Autodesk Inventor part; units mm, degrees
ref_plane "YZ Plane" through (0, 0, 0) normal (1, 0, 0) x (0, 1, 0)
ref_plane "XZ Plane" through (0, 0, 0) normal (0, 1, 0) x (-1, 0, 0)
ref_plane "XY Plane" through (0, 0, 0) normal (0, 0, 1) x (1, 0, 0)
sketch "スケッチ1" plane through (0, 0, 0) normal (0, 0, 1) x (1, 0, 0)
  circle A0 centre (0, 0) radius 13.5
  line L0 (0, 13.5) -> (14.5, 13.5)
  line L1 (14.5, 13.5) -> (14.5, -13.5)
  line L2 (14.5, -13.5) -> (0, -13.5)
  line L3 (0, -13.5) -> (0, 13.5)
  line L4 (0, 0) -> (14.5, 0) construction
  point P0 (0, 13.5)
  point P1 (0, -13.5)
  point P2 (0, -13.5)
  dimension "d0" = 27
  dimension "d1" = 27
  dimension "d2" = 14.5
extrude "プレート1" add sketch "スケッチ1" along normal blind 3
sketch "スケッチ2" plane through (17.5, 13.5, 6) normal (1, 0, 0) x (0, 1, 0)
  line L0 (-27, 0) -> (0, 0)
  line L1 (0, 0) -> (0, 19)
  line L2 (0, 19) -> (-27, 19)
  line L3 (-27, 19) -> (-27, 0)
edge flange "フランジ1" height 25 angle 90 thickness 3 bend radius 3 thickness toward (1, 0, 0) relief tear relief width 3 relief depth 1.5 edges at (14.5, 0, 3) wall of the first edge with corners at (17.5, -13.5, 6) (17.5, 13.5, 6) (17.5, 13.5, 25) (17.5, -13.5, 25)
bend "曲げ1"
corner "コーナー1"
sketch "スケッチ3" plane through (0, 0, 0) normal (0, 0, -1) x (-1, 0, 0)
  point P0 (0, 0)
  point P1 (10, 0)
  point P2 (-5, 8.6603)
  point P3 (-5, -8.6603)
  dimension "d14" = 10
  dimension "d17" = 360
hole "穴1" at (-10, 0, 0) at (5, 8.6603, 0) at (5, -8.6603, 0) direction (0, 0, 1) diameter 2.7 depth 3
sketch "スケッチ4" plane through (20.5, -13.5, 25) normal (1, 0, 0) x (0, 0, -1)
  circle A0 centre (-2, 14.5) radius 21
  line L0 (25, 27) -> (25, 0)
  point P0 (25, 13.5)
  dimension "d26" = 42
  dimension "d29" = 27
extrude "押し出し1" add sketch "スケッチ4" against normal up to surface (3 mm away)
sketch "スケッチ5" plane through (20.5, -13.5, 6) normal (1, 0, 0) x (0, 0, -1)
  arc A0 (-4.1255, 27) -> (-5.8095, 0) centre (-21, 14.5) ccw
  circle A1 centre (-21, 14.5) radius 14.5
  point P0 (6, 13.5)
  dimension "d30" = 29
extrude "押し出し2" cut sketch "スケッチ5" against normal up to surface (3 mm away)
sketch "スケッチ7" plane through (20.5, -13.5, 6) normal (1, 0, 0) x (0, 0, -1)
  circle A0 centre (-21, 14.5) radius 14.5
  point P0 (6, 13.5)
  point P1 (-39.5, 14.5)
  point P2 (-11.75, -1.5215)
  point P3 (-11.75, 30.5215)
  dimension "d33" = 18.5
  dimension "d36" = 360
hole "穴2" at (20.5, 1, 45.5) at (20.5, -15.0215, 17.75) at (20.5, 17.0215, 17.75) direction (-1, 0, 0) diameter 2.7 depth 3
fillet "フィレット1" radius 10 2 edges at (19, -13.5, 11.8095) (19, 13.5, 10.1255)
sketch "スケッチ9" plane through (0, 0, 0) normal (0, 0, -1) x (-1, 0, 0)
  arc A0 (0, -13.5) -> (0, 13.5) centre (0, 0) ccw
  line L0 (0, 13.5) -> (13.5, 13.5)
  line L1 (13.5, 13.5) -> (13.5, -13.5)
  line L2 (13.5, -13.5) -> (0, -13.5)
  line L3 (0, -13.5) -> (0, 13.5)
  circle A1 centre (-5, -8.6603) radius 1.35
  circle A2 centre (-5, 8.6603) radius 1.35
  circle A3 centre (10, 0) radius 1.35
  line L4 (0, 13.5) -> (-14.5, 13.5)
  line L5 (-14.5, 13.5) -> (-14.5, -13.5)
  line L6 (-14.5, -13.5) -> (0, -13.5)
  arc A4 (0, -13.5) -> (0, 13.5) centre (0, 0) ccw
  point P0 (13.5, 0)
  dimension "d48" = 13.5
  dimension "d49" = 27
extrude "押し出し3" add sketch "スケッチ9" against normal up to surface (3 mm away) contours A0 L1 L2 | A0 L0 L1
fillet "フィレット2" radius 6 2 edges at (-13.5, 13.5, 1.5) (-13.5, -13.5, 1.5)
equation "\"d24\" = Thickness"
equation "\"d3\" = Thickness"
equation "\"d4\" = BendReliefWidth"
equation "\"d5\" = BendReliefDepth"
equation "\"d6\" = MinimumRemnant"
equation "\"d7\" = TransitionRadius"
equation "\"d10\" = BendRadius"
equation "\"d11\" = CornerReliefSize"
equation "\"d12\" = GapSize"
equation "\"d13\" = JacobiRadiusSize"
equation "\"BendRadius\" = Thickness"
equation "\"BendReliefWidth\" = Thickness"
equation "\"BendReliefDepth\" = 0.5 * Thickness"
equation "\"CornerReliefSize\" = 4 * Thickness"
equation "\"MinimumRemnant\" = 2 * Thickness"
equation "\"TransitionRadius\" = BendRadius"
equation "\"JacobiRadiusSize\" = BendRadius"
equation "\"GapSize\" = Thickness"
properties part number "wrist_roll_plate" material "アルミニウム 6061"
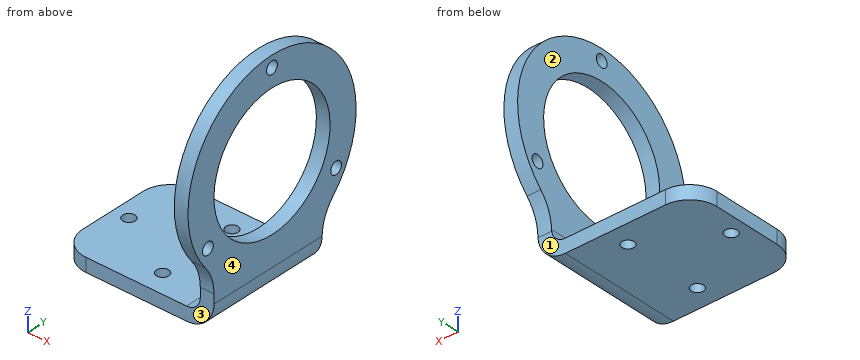
Source: CAD feature listing. Evaluate the final solid. Frame: model axes, mm. Face numbers are marked on the shaded views. A direction names the side the tool comes from. Round coordinates to 2 decimals unless told otherwise and drop trailing zeros. Loops run counter-clockwise (first coordinate to the right, second up) from the corner with the lowest first, then second, coordinate; pieces in that order, holes last. Notation, with made-up numbers: (75, 20) - (121, 20) arc R7 cw to (121, 30) - close; hole circle Ø9 at (-40, 6.25). An arc over 180 degrees is marked (long way). Write item = value, one per line. Start each with the question number.
(1) Section query D-D, the plane x = -10. Output: boundary loops of the cut face in (y, z).
(2) Section query C-C, the plane z = 17.75. Output: boundary loops of the cut face in (x, y), plus the area to 3 significant figures.
(3) Ray query, line 1 along Y through (x, z) = (5, 2.05); line 2 along Z through (x, y) = (-6, -1); line 3 along Y through (x, z) = (19, 17). Return the intervals inside material, ascending. Write a range as from..to.
(4) Section query A-A, the plane x = 5. Output: boundary loops of the cut face in (y, z).
(5) Set-up query: the marked faces 1, 2, 3 and 4. Return all of +Z, -Z, +X, -X, +Y, -Y with unobstructed straight access to the full face (end or side cutting, diameter ignored); none if empty.
(6) Pin query (flat end, axial travel): pin 1 (1 mm diameter, centred on x = -7.5, y = -4, fed in from +Z); pin 2 (5 mm diameter, centred on x = -9, y = 5, fed in from -Z); pin 3 (1.6 mm diameter, centred on x = -10, y = 0, fed in from -Z); pin 4 (1.7 mm diameter, centred on x = 10, z = 3.5, fed in from +Y). Return the tip coordinate at first contact, or that it passes through.
(7) Section query B-B, the plane z = 37. Output: boundary loops of the cut face in (x, y), plus the area to 3 significant figures.
Conclusion:
q1.outline = (-12.95, 0) - (-1.35, 0) - (-1.35, 3) - (-12.95, 3) - close; (1.35, 0) - (12.95, 0) - (12.95, 3) - (1.35, 3) - close
q2.outline = (17.5, -17.85) - (20.5, -17.85) - (20.5, -16.37) - (17.5, -16.37) - close; (17.5, -13.67) - (20.5, -13.67) - (20.5, -10.17) - (17.5, -10.17) - close; (17.5, 12.17) - (20.5, 12.17) - (20.5, 15.67) - (17.5, 15.67) - close; (17.5, 18.37) - (20.5, 18.37) - (20.5, 19.85) - (17.5, 19.85) - close
q2.area = 29.9 mm2
q3.line_1 = -13.5..-10.01, -7.31..7.31, 10.01..13.5
q3.line_2 = 0..3
q3.line_3 = -17.47..-16.14, -13.9..-9.5, 11.5..15.9, 18.14..19.47
q4.outline = (-13.5, 0) - (-10.01, 0) - (-10.01, 3) - (-13.5, 3) - close; (-7.31, 0) - (7.31, 0) - (7.31, 3) - (-7.31, 3) - close; (10.01, 0) - (13.5, 0) - (13.5, 3) - (10.01, 3) - close
q5.face_1 = -Z, +X, -X, +Y
q5.face_2 = +Z, -X, +Y, -Y
q5.face_3 = -Z, +X, -X, -Y
q5.face_4 = +Z, -Z, +X, +Y, -Y
q6.pin_1 = 3
q6.pin_2 = 0
q6.pin_3 = through
q6.pin_4 = 13.5
q7.outline = (17.5, -17.47) - (20.5, -17.47) - (20.5, -9.5) - (17.5, -9.5) - close; (17.5, 11.5) - (20.5, 11.5) - (20.5, 19.47) - (17.5, 19.47) - close
q7.area = 47.8 mm2
